Model file for the job. Use its own axes, mm. Face numbers are marked on the shaded views. Round coordinates to 2 decimals unless told otherwise and drop trailing zeros. Order: outer loops, then holes, each group sorted by start corner. A loop starts at its lowest first (then second) coordinate and runs counter-clockwise, first axis right, second up. Notation, with made-up numbers: (55.25, 85.25) - (106.25, 85.25) arc R23 cw to (106.25, 121.25) - close; hole circle Ø2 at (76, 87). An arc over 180 degrees is marked (long way). Answer as CSV lines item,"result". Start each with the question number.
1. Pin check, flat tips, straight feed: pin 1 Ø4 at (y, z) = (-21.5, -105) entering from +X; pin 2 Ø4 at (x, z) = (-63, -46.5) entering from +Y; pin 3 Ø8 at (x, z) = (-66.5, -176) entering from -Y. Stop position of each tip, or through.
2. Pull direction X, two halves, no side cores. Call the marked faces 1, 2 and 3: released by +X, released by -X, zero draft, split by the parting line, or undercut.
3. Band-saw the part on A-A on y = 0. List the corners of the cut face in (x, z) (3 decimals).
4. Band-saw the part on C-C on z = -203.2. List the corners of the cut face in (x, y) (3 decimals), then the cut area to 3 significant figures.
5. Wall check: line 1 along Y through (x, z) = (0, 251); line 2 along X through (y, z) = (4.5, -87); line 3 along Z through (x, y) = (-10.5, -31.5). Give the ranges that are in metal, low to high. Write a range as [from, to].
6. Band-saw the part on B-B on z = 182.5. List the corners of the cut face in (x, y), then the cut area to 3 significant figures.
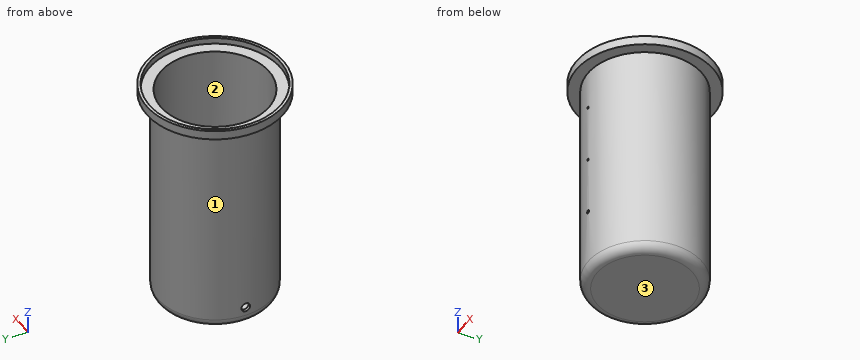
```python
from build123d import *

# Parameters (mm, degrees)
F2_T     = -6.35
F4_DEPTH = 150.001
F6_DEPTH = 150.001


with BuildPart() as f1:
    # F0 (on Front) → F1 (revolve)
    with BuildSketch(Plane.XZ):
        with BuildLine():
            Line((0, 257.5), (0, -242.5))
            Line((0, -242.5), (105, -242.5))
            ThreePointArc((105, -242.5), (119.1421356237, -236.6421356237), (125, -222.5))
            Line((125, -222.5), (125, 237.5))
            Line((125, 237.5), (150, 237.5))
            Line((150, 237.5), (150, 257.5))
            Line((150, 257.5), (0, 257.5))
        make_face()
    revolve(axis=Axis((0, 0, 7.5), (0, 0, -1)))

    # F2
    f2_openings = [f1.faces().sort_by_distance(p)[0] for p in [
        (0, 0, 257.5),
    ]]
    offset(amount=F2_T, openings=f2_openings, kind=Kind.INTERSECTION)

    # F3 (on Front) → F4 (cut, through all)
    with BuildSketch(Plane.XZ):
        with BuildLine():
            ThreePointArc((0, 149.86), (1.7960512242, 150.6039487758), (2.54, 152.4))
            ThreePointArc((2.54, 152.4), (1.7960512242, 154.1960512242), (0, 154.94))
            Line((0, 154.94), (0, 149.86))
        make_face()
        with BuildLine():
            ThreePointArc((3.81, -101.6), (2.6940768363, -98.9059231637), (0, -97.79))
            Line((0, -97.79), (0, -105.41))
            ThreePointArc((0, -105.41), (2.6940768363, -104.2940768363), (3.81, -101.6))
        make_face()
        with BuildLine():
            Line((0, -105.41), (0, -97.79))
            ThreePointArc((0, -97.79), (-3.81, -101.6), (0, -105.41))
        make_face()
        with BuildLine():
            ThreePointArc((2.54, 25.4), (1.7960512242, 27.1960512242), (0, 27.94))
            Line((0, 27.94), (0, 22.86))
            ThreePointArc((0, 22.86), (1.7960512242, 23.6039487758), (2.54, 25.4))
        make_face()
        with BuildLine():
            Line((0, 22.86), (0, 27.94))
            ThreePointArc((0, 27.94), (-2.54, 25.4), (0, 22.86))
        make_face()
        with BuildLine():
            Line((0, 149.86), (0, 154.94))
            ThreePointArc((0, 154.94), (-2.54, 152.4), (0, 149.86))
        make_face()
    extrude(amount=F4_DEPTH, mode=Mode.SUBTRACT)

    # F5 (on Right) → F6 (cut, through all)
    with BuildSketch(Plane.YZ):
        with BuildLine():
            ThreePointArc((0, -193.675), (-6.7351920908, -209.9351920908), (9.525, -203.2))
            ThreePointArc((9.525, -203.2), (6.7351920908, -196.4648079092), (0, -193.675))
        make_face()
    extrude(amount=-F6_DEPTH, mode=Mode.SUBTRACT)


solid = f1.part
```
Reply:
1,pin 1,"stops at x = 123.47"
1,pin 2,"stops at y = 109.11"
1,pin 3,"stops at y = -108.25"
2,face 1,"split by the parting line"
2,face 2,"undercut"
2,face 3,"zero draft"
3,outline,"(-150, 237.5) - (-125, 237.5) - (-125, -193.675) - (-118.65, -193.675) - (-118.65, 243.85) - (-143.65, 243.85) - (-143.65, 257.5) - (-150, 257.5) - close; (-125, -222.5) arc R20 ccw to (-105, -242.5) - (105, -242.5) arc R20 ccw to (125, -222.5) - (125, 237.5) - (150, 237.5) - (150, 257.5) - (143.65, 257.5) - (143.65, 243.85) - (118.65, 243.85) - (118.65, -222.5) arc R13.65 cw to (105, -236.15) - (-105, -236.15) arc R13.65 cw to (-118.65, -222.5) - (-118.65, -212.725) - (-125, -212.725) - close"
4,outline,"(-124.637, -9.525) arc R125 ccw (long way) to (-124.637, 9.525) - (-118.267, 9.525) arc R118.65 cw (long way) to (-118.267, -9.525) - close"
4,area,"4,740 mm2"
5,line 1,"y = [-150, -143.65], [143.65, 150]"
5,line 2,"x = [-124.92, -118.56], [118.56, 124.92]"
5,line 3,"z = [-242.5, -236.15]"
6,outline,"circle Ø250 at (0, 0); hole circle Ø237.3 at (0, 0)"
6,area,"4,860 mm2"
